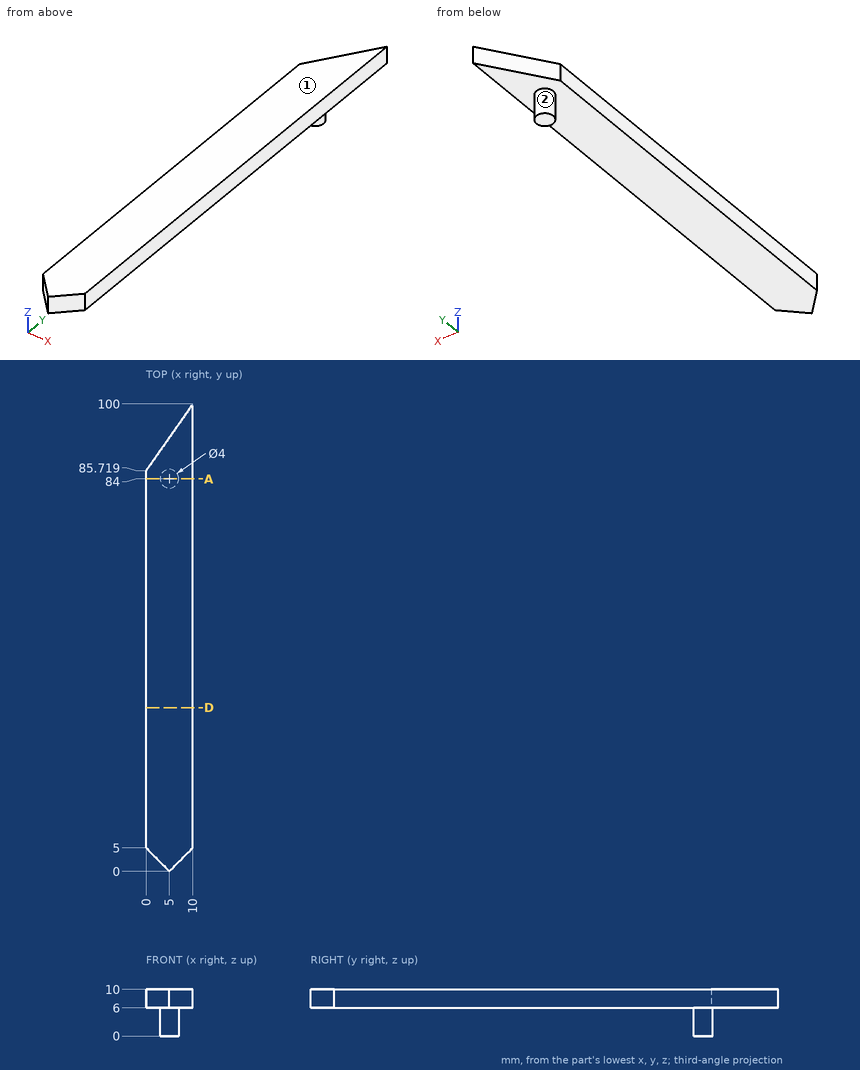
The figure shows three views and two pictorial views of one solid part (mm, origin at its lowest corner). Answer the questions. A direction names the side the tool comes from. Give positions to 0.01 mm unless a question says otherwise; leave off trailing zeros. Write each loop counter-clockwise with the first axis right and the second up, starting at its lowest first coordinate (ties: lowest second). Pieces come first, ordered by that corner, then holes. Notation, with made-up numbers: (-23, -27.75) -> (33, -27.75) arc R15 cw to (33, -4.75) -> close; hole circle Ø5 at (18, -27.5). An arc over 180 degrees is marked (long way). Use one line per item in the form item = value.
1) Each of these flat-tipped pins is pushed along its axis until it touches: P1, Ø3, axis at x = 7.5, z = 8.5, coming from the -Y side; P2, Ø1.5, axis at x = 3.5, y = 41.5, coming from the -Z side. Where does it stop, or does it pass through?
Result:
P1 = 1
P2 = 6
2) Section D-D on y = 35 is taken. Write down the section's boundary in (x, z).
Result:
outline = (0, 6) -> (10, 6) -> (10, 10) -> (0, 10) -> close
3) Straight lines are drawn through the part: probe 1 along Z at (x, y) = (7, 27.5); probe 2 along Y at (x, z) = (8.25, 8); probe 3 along Y at (x, z) = (3, 8) (1 decimal). For each, find the intervals that lie inside material, in ascending order.
Result:
probe_1 = 6 to 10
probe_2 = 3.25 to 97.5
probe_3 = 2 to 90
4) A tool of negligible diameter and unlimited length cuts with its end or side. For the marked faces 1 and 2, from which of +Z, -Z, +X, -X, +Y, -Y can it reach the whole face along a straight path? Write none if from no direction.
Result:
face_1 = +Z, +X, -X, +Y, -Y
face_2 = -Z
5) Section A-A on y = 84 is taken. Write down the section's boundary in (x, z), plus the area to 3 significant figures.
Result:
outline = (0, 6) -> (3, 6) -> (3, 0) -> (7, 0) -> (7, 6) -> (10, 6) -> (10, 10) -> (0, 10) -> close
area = 64.0 mm²
